Autodesk Fusion 360 part; units mm, degrees
sketch "草图1" plane through (0, 0, 0) normal (0, 1, 0) x (1, 0, 0)
  line L0 (28, 3) -> (28, 5)
  line L1 (28, 5) -> (0, 5)
  arc A0 (0, 5) -> (5, 0) centre (0, 0) ccw
  line L2 (28, 3) -> (0, 3)
  arc A1 (0, 3) -> (3, 0) centre (0, 0) ccw
  line L3 (3, 0) -> (5, 0)
  line L4 (0, 3) -> (0, 5)
  dimension "d1" = 2
  dimension "d2" = 3
  dimension "d3" = 5
  dimension "d4" = 2
  dimension "d5" = 28
extrude "拉伸1" add sketch "草图1" along normal mid plane 16 contours A0 A1 L3 L4
extrude "拉伸2" add sketch "草图1" along normal mid plane 45 contours L0 L1 L2 L4
sketch "草图2" plane through (0, 0, -3) normal (0, 0, 1) x (-1, 0, 0)
  line L0 (-28, 22.5) -> (-28, -22.5)
  line L1 (-28, -22.5) -> (0, -22.5)
  line L2 (0, -22.5) -> (0, -8)
  line L3 (0, -8) -> (0, 8)
  line L4 (0, 8) -> (0, 22.5)
  line L5 (0, 22.5) -> (-28, 22.5)
  line L6 (0, -8) -> (-18.4849, -21.3625)
  arc A0 (-28, -16.5) -> (-18.4849, -21.3625) centre (-22, -16.5) ccw
  line L7 (-28, -16.5) -> (-28, 16.5)
  arc A1 (-18.4849, 21.3625) -> (-28, 16.5) centre (-22, 16.5) ccw
  line L8 (-18.4849, 21.3625) -> (0, 8)
  line L9 (0, 8) -> (0, -8)
  line L10 (10, 0) -> (-55, 0) construction
  circle A2 centre (-22, -16.5) radius 2
  circle A3 centre (-22, 16.5) radius 2
  line L11 (-22, -16.5) -> (-22, 16.5) construction
  circle A4 centre (-22, -5.5) radius 2
  circle A5 centre (-22, 5.5) radius 2
  circle A6 centre (-22, 16.5) radius 2
  line L12 (-12, 2) -> (-22, 2)
  arc A7 (-22, 2) -> (-22, -2) centre (-22, 0) ccw
  line L13 (-22, -2) -> (-12, -2)
  arc A8 (-12, -2) -> (-12, 2) centre (-12, 0) ccw
  dimension "d10" = 6
  dimension "d11" = 6
  dimension "d12" = 45
  dimension "d13" = 4
  dimension "d14" = 4
  dimension "d17" = 33
  dimension "d18" = 0
  dimension "d19" = 4
  dimension "d20" = 14
extrude "拉伸3" cut sketch "草图2" against normal blind 11 contours L0 L5 A1 | L4 L5 A1 L8 | L0 L1 A0 | L1 L2 L6 A0 | A2 | A3 A6 | A4 | A5 | L12 A7 L13 A8
Read the model definition and answer for the solid it produces. Units are mm, in the model's axes. A direction names the side the tool comes from. Coordinates: 2 decimals unless noted, no trailing zeros. Write each loop counter-clockwise with the first axis right and the second up, starting at its lowest first coordinate (ties: lowest second). Pieces come first, ordered by that corner, then holes. Notation, with made-up numbers: (75, 25) -> (127, 25) arc R17 cw to (127, 32) -> close; hole circle Ø7 at (81.25, -26). An arc over 180 degrees is marked (long way). Write item = value, one per line.
(1) Given pin 1 Ø6.5 at (x, y) = (22, -5.5) entering from +Z; pin 2 Ø0.6 at (x, z) = (16.5, -3.5) entering from -Y; pin 3 Ø1.6 at (x, z) = (17.5, -4.5) entering from +Y; pin 4 Ø5.5 at (x, z) = (0, 0) entering from +Y, each flat-ended and moving along its own axis, determine where each tip first touches the part or whether it passes through.
From the geometry:
pin_1 = -3
pin_2 = -20.14
pin_3 = 21.23
pin_4 = through
(2) For a pull along X with two mould halves and no side action, classify faces 1 (the face through (-2.3, -8, 2.2)), 2 (the face through (9.372, -14.775, -3.986)), 3 (the face through (-2.05, -0.11, 2.19)), 4 (the face through (24.648, -21.884, -3.986)) as +X half, -X half, draft (parallel to the pull), parting line (faces both ways), or undercut.
From the geometry:
face_1 = draft
face_2 = -X half
face_3 = undercut
face_4 = parting line
(3) Which of the six approach directions +Z, -Z, +X, -X, +Y, -Y give full straight-line access (tool end or side, diameter ignored) to faces 5 (the face through (10, 0, -4)), 6 (the face through (4, 0, 0)), 7 (the face through (-2.3, 8, 2.2))?
From the geometry:
face_5 = +Z, -Z
face_6 = +X, +Y, -Y
face_7 = +Z, -X, +Y
(4) Section D-D on y = 3 is taken. Write down the section's boundary in (x, z).
From the geometry:
outline = (0, -5) -> (28, -5) -> (28, -3) -> (0, -3) arc R3 cw (long way) to (3, 0) -> (5, 0) arc R5 ccw (long way) to start
(5) Section B-B on x = 11 is taken. Write down the section's boundary in (y, z), plus the area to 3 significant figures.
From the geometry:
outline = (-15.95, -5) -> (-1.73, -5) -> (-1.73, -3) -> (-15.95, -3) -> close; (1.73, -5) -> (15.95, -5) -> (15.95, -3) -> (1.73, -3) -> close
area = 56.9 mm2
(6) Section C-C on z = -4 is taken. Write down the section's boundary in (x, y).
From the geometry:
outline = (-3, -8) -> (0, -8) -> (18.48, -21.36) arc R6 ccw to (28, -16.5) -> (28, 16.5) arc R6 ccw to (18.48, 21.36) -> (0, 8) -> (-3, 8) -> close; hole (12, -2) -> (22, -2) arc R2 ccw to (22, 2) -> (12, 2) arc R2 ccw to start; hole circle Ø4 at (22, -16.5); hole circle Ø4 at (22, -5.5); hole circle Ø4 at (22, 5.5); hole circle Ø4 at (22, 16.5)
(7) Straight lines are drawn through the part: L1, parallel to Y at x = 22, z = -3.6; L2, parallel to X at y = 7, z = 0.25; L3, parallel to Z at x = 3, y = -9. For each, find the intervals that lie inside material, in ascending order. Write a range as from..to.
From the geometry:
L1 = -22.5..-18.5, -14.5..-7.5, -3.5..-2, 2..3.5, 7.5..14.5, 18.5..22.5
L2 = -4.99..-2.99, 2.99..4.99
L3 = -5..-3
(8) Section A-A on y = -5.5 is taken. Write down the section's boundary in (x, z), plus the area to 3 significant figures.
From the geometry:
outline = (0, -5) -> (20, -5) -> (20, -3) -> (0, -3) arc R3 cw (long way) to (3, 0) -> (5, 0) arc R5 ccw (long way) to start; (24, -5) -> (28, -5) -> (28, -3) -> (24, -3) -> close
area = 85.7 mm2
